Build history of the part. All positions in model axes, mm. A direction names the side the tool comes from. Round coordinates to 2 decimals unless told otherwise and drop trailing zeros. Write each loop counter-clockwise with the first axis right and the second up, starting at its lowest first coordinate (ties: lowest second). Pieces come first, ordered by that corner, then holes. Notation, with made-up numbers: (-37.75, 86.25) -> (-1.75, 86.25) arc R25 cw to (-1.75, 107.25) -> close; hole circle Ø1 at (77, 80). An arc over 180 degrees is marked (long way). One line per question, with ' | ' between items.
from build123d import *

# Parameters (mm, degrees)
F1_DEPTH = 12
F0_R     = 10
F2_DEPTH = 20
F5_DEPTH = 10
F4_R     = 6
F6_DEPTH = 12


# Not quite as in the source:
# - a pattern or mirror of a feature is missing from the dataset's text; its kind, count and spacing are read off the source's solid


with BuildPart() as f1:
    # F0 (on Front) → F1 (new body)
    with BuildSketch(Plane.XZ):
        with BuildLine():
            ThreePointArc((17.3264581055, 84.9896871582), (19.3200564454, 80.1706304205), (20, 75))
            ThreePointArc((20, 75), (-5.1706304205, 55.6799435546), (-17.3264581055, 84.9896871582))
            Line((-17.3264581055, 84.9896871582), (-37.5, 50))
            Line((-37.5, 50), (-37.5, 0))
            Line((-37.5, 0), (37.5, 0))
            Line((37.5, 0), (37.5, 50))
            Line((37.5, 50), (17.3264581055, 84.9896871582))
        make_face()
        with BuildLine():
            ThreePointArc((8, 20), (0, 12), (-8, 20))
            Line((-8, 20), (-8, 34))
            ThreePointArc((-8, 34), (0, 42), (8, 34))
            Line((8, 34), (8, 20))
        make_face(mode=Mode.SUBTRACT)
    extrude(amount=F1_DEPTH)

    # F0 (on Front) → F2 (join)
    with BuildSketch(Plane.XZ):
        with BuildLine():
            ThreePointArc((-17.3264581055, 84.9896871582), (-5.1706304205, 55.6799435546), (20, 75))
            ThreePointArc((20, 75), (19.3200564454, 80.1706304205), (17.3264581055, 84.9896871582))
            ThreePointArc((17.3264581055, 84.9896871582), (0, 95), (-17.3264581055, 84.9896871582))
        make_face()
        with Locations((0, 75)):
            Circle(F0_R, mode=Mode.SUBTRACT)
    extrude(amount=F2_DEPTH)

    # F4 (on offset) → F5 (join)
    with BuildSketch(Plane.YZ.offset(16.5)):
        with BuildLine():
            ThreePointArc((-40.6341440633, 20.3337600333), (-27.5061001769, 23.1267634279), (-20, 12))
            ThreePointArc((-20, 12), (-23.5147186258, 3.5147186258), (-32, 0))
            Line((-32, 0), (-12, 0))
            Line((-12, 0), (-12, 50))
            Line((-12, 50), (-40.6341440633, 20.3337600333))
        make_face()
    f5 = extrude(amount=F5_DEPTH)

    # F5_copies: F5 across plane
    add(f5.mirror(Plane(origin=(0, 0, 0), x_dir=(0, 0, -1), z_dir=(-1, 0, 0))))

    # F4 (on offset) → F6 (join)
    with BuildSketch(Plane.YZ.offset(16.5)):
        with BuildLine():
            ThreePointArc((-32, 0), (-23.5147186258, 3.5147186258), (-20, 12))
            ThreePointArc((-20, 12), (-27.5061001769, 23.1267634279), (-40.6341440633, 20.3337600333))
            ThreePointArc((-40.6341440633, 20.3337600333), (-43.0454769114, 7.3098571664), (-32, 0))
        make_face()
        with Locations((-32, 12)):
            Circle(F4_R, mode=Mode.SUBTRACT)
    f6 = extrude(amount=F6_DEPTH)

    # F6_copies: F6 across plane
    add(f6.mirror(Plane(origin=(0, 0, 0), x_dir=(0, 0, -1), z_dir=(-1, 0, 0))))


solid = f1.part
(1) Slice it at B-B (x = 0). Write the cut outline in (y, z).
Calculated:
outline: (-20, 55) -> (-12, 55) -> (-12, 42) -> (0, 42) -> (0, 65) -> (-20, 65) -> close; (-20, 85) -> (0, 85) -> (0, 95) -> (-20, 95) -> close; (-12, 0) -> (0, 0) -> (0, 12) -> (-12, 12) -> close
(2) Slice it at D-D (z = 36). Write the cut outline in (x, y), then the cut area to 3 significant figures.
Calculated:
outline: (-37.5, -12) -> (-26.5, -12) -> (-26.5, -25.51) -> (-16.5, -25.51) -> (-16.5, -12) -> (-7.75, -12) -> (-7.75, 0) -> (-37.5, 0) -> close; (7.75, -12) -> (16.5, -12) -> (16.5, -25.51) -> (26.5, -25.51) -> (26.5, -12) -> (37.5, -12) -> (37.5, 0) -> (7.75, 0) -> close | area: 984 mm2
(3) Slice it at A-A (y = -17.5). Write the cut outline in (x, z), then the cut area to 3 significant figures.
Calculated:
outline: (-26.5, 0) -> (-16.5, 0) -> (-16.5, 44.3) -> (-26.5, 44.3) -> close; circle Ø40 at (0, 75); (16.5, 0) -> (26.5, 0) -> (26.5, 44.3) -> (16.5, 44.3) -> close; hole circle Ø20 at (0, 75) | area: 1,830 mm2
(4) Mould opens along X. For faces 1 (the flat face through (-28.5, -38, 10)), 2 (the cylindrical face through (22.42, -36.76, 8.35)), 3 (the flat face through (-16.5, -25, 20)), 4 (the flat face through (16.5, -25, 20)) say: pulls with the +X half, pulls with the -X half, needs draft (parallel to the pull), parting line crosses it, or undercut.
Calculated:
face 1: pulls with the -X half | face 2: needs draft | face 3: undercut | face 4: undercut
(5) Slice it at C-C (y = -3.5). Write the cut outline in (x, z), then the cut area to 3 significant figures.
Calculated:
outline: (-37.5, 0) -> (37.5, 0) -> (37.5, 50) -> (17.33, 84.99) arc R20 ccw to (-17.33, 84.99) -> (-37.5, 50) -> close; hole circle Ø20 at (0, 75); hole (-8, 20) arc R8 ccw to (8, 20) -> (8, 34) arc R8 ccw to (-8, 34) -> close | area: 5,180 mm2
(6) 3-axis set-ups, long thin cutter, end or side, ignore diameter. For faces 5 (the flat face through (28.5, -38, 10)), 6 (the cylindrical face through (0, -6, 12)), 7 (the cylindrical face through (-22.42, -36.76, 8.35)), 8 (the flat face through (-5, -20, 84)), 9 (the flat face through (-1, -9, 0)): which of +Z, -Z, +X, -X, +Y, -Y reach the whole face in a straight line?
Calculated:
face 5: +Z, -Z, +X, -Y | face 6: +Y, -Y | face 7: +X, -X | face 8: +Z, +X, -X, -Y | face 9: -Z, +X, -X, +Y, -Y
(7) Drop flat-ended pins along their axis: pin 1 (20 mm diameter, centred on x = 7.5, z = 83.5, fed in from -Y); pin 2 (23 mm diameter, centred on y = -20.5, z = 21, fed in from -X); pin 3 (7 mm diameter, centred on y = -31.5, z = 8, fed in from -X); pin 4 (10 mm diameter, centred on x = -5.5, y = -17, fed in from +Z). Give the stop position or say it passes through.
Calculated:
pin 1: y = -20 | pin 2: x = -37.5 | pin 3: x = -28.5 | pin 4: z = 94.99
(8) Wall check: line 1 (Z direction, x = 0, y = -10); line 2 (X direction, y = -42, z = 7); line 3 (Y direction, x = 22, z = 71). Give the ranges that are in metal, low to high. Write a range as from..to.
Calculated:
line 1: 0..12, 42..65, 85..95 | line 2: -28.5..-16.5, 16.5..28.5 | line 3: -12..0
